```python
from build123d import *

# Parameters (mm, degrees)
EXTRUDE_1_DEPTH = 54


with BuildPart() as part:
    # 草图1 → 凸台-拉伸1 (new body)
    with BuildSketch(Plane(origin=(0, 0, 0), x_dir=(1, 0, 0), z_dir=(0, 1, 0))):
        with BuildLine():
            ThreePointArc((-224.091230242, 162.375487068), (-244.806924848, 157.652626052), (-246.078397413, 136.443458772))
            Line((-246.078397413, 136.443458772), (-197.199257089, 62.405433085))
            ThreePointArc((-197.199257089, 62.405433085), (-195.041572593, 59.971891729), (-192.288857087, 58.239759155))
            Line((-192.288857087, 58.239759155), (213.190233659, -122.721502411))
            ThreePointArc((213.190233659, -122.721502411), (218.617938967, -123.695981456), (223.875273721, -122.031642066))
            Line((223.875273721, -122.031642066), (274.861498447, -90.862018276))
            ThreePointArc((274.861498447, -90.862018276), (283.435193918, -74.339940028), (272.79992067, -59.063216341))
            Line((272.79992067, -59.063216341), (-224.091230242, 162.375487068))
        make_face()
        with BuildLine():
            ThreePointArc((-245.243860787, 136.994411239), (-244.044186993, 157.005918262), (-224.498286741, 161.462084086))
            Line((-224.498286741, 161.462084086), (272.392864172, -59.976619323))
            ThreePointArc((272.392864172, -59.976619323), (282.437288906, -74.404636139), (274.33990985, -90.008821151))
            Line((274.33990985, -90.008821151), (222.246746967, -121.767406417))
            ThreePointArc((222.246746967, -121.767406417), (217.926670991, -122.719757656), (213.59777898, -121.808317429))
            Line((213.59777898, -121.808317429), (-191.881311765, 59.152944137))
            ThreePointArc((-191.881311765, 59.152944137), (-194.280273175, 60.63880571), (-196.19690286, 62.709875751))
            Line((-196.19690286, 62.709875751), (-245.243860787, 136.994411239))
        make_face(mode=Mode.SUBTRACT)
    extrude(amount=EXTRUDE_1_DEPTH)


solid = part.part
```
CAD build for the part. Positions are in the model's coordinates, mm. A direction names the side the tool comes from. Round coordinates to 2 decimals unless told otherwise and drop trailing zeros. Order: outer loops, then holes, each group sorted by start corner. A loop starts at its lowest first (then second) coordinate and runs counter-clockwise, first axis right, second up.
Q1. Slice it at B-B (y = 48). Write the cut outline in (x, z).
Q2. Wall check: L1, parallel to Z at x = -177, y = 16.5; L2, parallel to Z at x = 206.5, y = 43.5; L3, parallel to X at y = 12, z = -87.5. Give the ranges that are in metal, low to high.
Q3. Drop flat-ended pins along their axis: pin 1 (12 mm diameter, centred on x = 103, y = 30, fed in from +Z); pin 2 (3 mm diameter, centred on x = -23, y = 39, fed in from -Z); pin 3 (1 mm diameter, centred on x = -116, y = 39.5, fed in from +Z). Give the stop position or say it passes through.
Q4. Slice it at C-C (x = -94). Write the cut outline in (y, z), and give its area (3 significant figures).
Q5. Slice it at A-A (z = 67). Write the cut outline in (x, y).
Q6. Two-plate mould, pull along X, no slides. Class faces 1 (the flat face through (20.469, 26.622, -52.293)), 2 (the cylindrical face through (-244.6, 26.62, -157.89)), 3 (the flat face through (27.833, 26.622, -50.106)): pulls with the +X half, pulls with the -X half, needs draft (parallel to the pull), parting line crosses it, or undercut.
Q7. Which spindle directions (+Z, -Z, +X, -X, +Y, -Y) get a long thin tool onto all of the face, cutting with end or side? Do faces 4 (the cylindrical face through (282.42, 26.62, 74.15)), 5 (the flat face through (249.011, 26.622, 106.665)). Say none if no direction does.
Results below:
1. outline: (-246.08, -136.44) arc R17.71 ccw to (-224.09, -162.38) - (272.8, 59.06) arc R18 ccw to (274.86, 90.86) - (223.88, 122.03) arc R11.5 ccw to (213.19, 122.72) - (-192.29, -58.24) arc R11.5 ccw to (-197.2, -62.41) - close; hole (-245.24, -136.99) arc R16.71 ccw to (-224.5, -161.46) - (272.39, 59.98) arc R17 ccw to (274.34, 90.01) - (222.25, 121.77) arc R10.5 ccw to (213.6, 121.81) - (-191.88, -59.15) arc R10.5 ccw to (-196.2, -62.71) - close
2. L1: z = -141.39 to -140.29, -52.51 to -51.42
2. L2: z = 29.52 to 30.61, 118.64 to 119.74
2. L3: x = -213.77 to -212.56, -58.53 to -56.08
3. pin 1: stops at z = 76.22
3. pin 2: stops at z = -73.43
3. pin 3: stops at z = -23.97
4. outline: (0, -104.4) - (54, -104.4) - (54, -103.31) - (0, -103.31) - close; (0, -15.47) - (54, -15.47) - (54, -14.37) - (0, -14.37) - close
4. area: 118 mm2
5. outline: (88.34, 0) - (90.79, 0) - (90.79, 54) - (88.34, 54) - close; (280.19, 0) - (281.34, 0) - (281.34, 54) - (280.19, 54) - close
6. face 1: undercut
6. face 2: parting line crosses it
6. face 3: pulls with the +X half
7. face 4: +Y, -Y
7. face 5: +Z, +X, +Y, -Y
